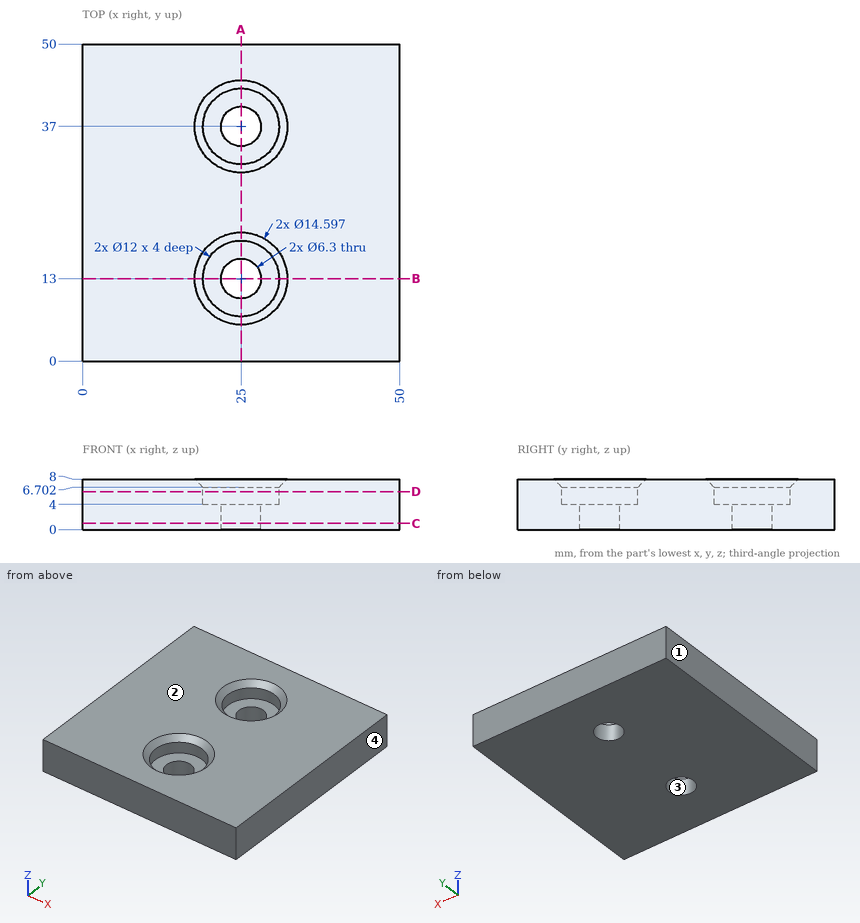
Geometry: see drawing. Coordinates: mm, zero at the bounding-box minimum. Give positions to 0.01 mm unless a question says otherwise; leave off trailing zeros. Order: outer loops, then holes, each group sorted by start corner. A loop starts at its lowest first (then second) coordinate and runs counter-clockwise, first axis right, second up. Notation, with made-up numbers: M -6.5,-27 L 26.5,-27 A23 ccw 26.5,-14 Z; hole C -36.5,31.25 d9. An arc over 180 degrees is marked long. Answer as CSV lines item,"result". Start each with the question number.
1) Mould query, pull axis X, two halves, no side actions, for the marked faces 1, 2, 3 and 4. Classes: +X half, -X half, draft (parallel to the pull), parting line (faces both ways), or undercut.
2) Cut plane A-A (x = 25). Output: boundary loops of the cut face in (y, z), then the cut area to 3 significant figures.
3) Cut plane B-B (y = 13). Output: boundary loops of the cut face in (x, z).
4) First-contact query: P1, Ø7, axis at x = 25, y = 37, coming from the +Z side; P2, Ø9.5, axis at x = 25, y = 11, coming from the +Z side. Flat tips, straight axial feed; report the tip coordinate or a pass-through.
5) Line query: line 1 (Y direction, x = 25, z = 5.25); line 2 (Y direction, x = 25, z = 2.7); line 3 (X direction, y = 37, z = 6.5). Output: solid intervals per line, ascending. Write a range as from..to.
6) Cut plane C-C (z = 1). Output: boundary loops of the cut face in (x, y), then the cut area to 3 significant figures.
7) Cut plane D-D (z = 6). Output: boundary loops of the cut face in (x, y), then the cut area to 3 significant figures.
Findings below:
1,face 1,"-X half"
1,face 2,"draft"
1,face 3,"undercut"
1,face 4,"+X half"
2,outline,"M 0,0 L 9.85,0 L 9.85,4 L 7,4 L 7,6.7 L 5.7,8 L 0,8 Z; M 16.15,0 L 33.85,0 L 33.85,4 L 31,4 L 31,6.7 L 29.7,8 L 20.3,8 L 19,6.7 L 19,4 L 16.15,4 Z; M 40.15,0 L 50,0 L 50,8 L 44.3,8 L 43,6.7 L 43,4 L 40.15,4 Z"
2,area,"250 mm²"
3,outline,"M 0,0 L 21.85,0 L 21.85,4 L 19,4 L 19,6.7 L 17.7,8 L 0,8 Z; M 28.15,0 L 50,0 L 50,8 L 32.3,8 L 31,6.7 L 31,4 L 28.15,4 Z"
4,P1,"stops at z = 4"
4,P2,"stops at z = 7.45"
5,line 1,"y = 0..7, 19..31, 43..50"
5,line 2,"y = 0..9.85, 16.15..33.85, 40.15..50"
5,line 3,"x = 0..19, 31..50"
6,outline,"M 0,0 L 50,0 L 50,50 L 0,50 Z; hole C 25,13 d6.3; hole C 25,37 d6.3"
6,area,"2,440 mm²"
7,outline,"M 0,0 L 50,0 L 50,50 L 0,50 Z; hole C 25,13 d12; hole C 25,37 d12"
7,area,"2,270 mm²"
